Check sheet for the modelled part. Datum: model origin and axes. Units: mm. A direction names the side the tool comes from. Round coordinates to 2 decimals unless told otherwise and drop trailing zeros. Loops run counter-clockwise (first coordinate to the right, second up) from the corner with the lowest first, then second, coordinate; pieces in that order, holes last. Notation, with made-up numbers: (-24, -11.75) - (-5, -11.75) arc R34 ccw to (-5, 22.25) - close; hole circle Ø5 at (-33.75, 3.5). An arc over 180 degrees is marked (long way). Put each result on its own line as item: value.
```python
from build123d import *

# Parameters (mm, degrees)
EXTRUDE_1_DEPTH     = 10
SKETCH_2_W          = 16
SKETCH_2_H          = 40
CUT_EXTRUDE_1_DEPTH = 10
SKETCH_3_R          = 2
CUT_EXTRUDE_2_DEPTH = 50


with BuildPart() as part:
    # 草图1 → 凸台-拉伸1 (new, symmetric)
    with BuildSketch(Plane.XY):
        Polygon((0, 42), (0, 2), (0, 0), (7, 0), (7, 44), (0, 44), align=None)
    extrude(amount=EXTRUDE_1_DEPTH, both=True)

    # 草图2 → 切除-拉伸1 (cut, symmetric)
    with BuildSketch(Plane(origin=(7, 0, 0), x_dir=(0, 0, -1), z_dir=(1, 0, 0))):
        with Locations((0, 22)):
            Rectangle(SKETCH_2_W, SKETCH_2_H)
    extrude(amount=CUT_EXTRUDE_1_DEPTH, both=True, mode=Mode.SUBTRACT)

    # 草图3 → 切除-拉伸2 (cut)
    with BuildSketch(Plane(origin=(0, 44, 0), x_dir=(1, 0, 0), z_dir=(0, 1, 0))):
        with Locations(Location((4, 5, 0), (0, 0, 270))):
            Circle(SKETCH_3_R)
        with Locations(Location((4, -5, 0), (0, 0, 270))):
            Circle(SKETCH_3_R)
    extrude(amount=-CUT_EXTRUDE_2_DEPTH, mode=Mode.SUBTRACT)


solid = part.part
```
Item 1: Section check C-C on z = -1.5. Enter the section's corners in (x, y).
Filled sheet:
outline: (0, 0) - (7, 0) - (7, 2) - (0, 2) - close; (0, 42) - (7, 42) - (7, 44) - (0, 44) - close
Item 2: Release check for a two-part mould opening along Y. For faces 1 (the flat face through (4, 44, 0)), 2 (the flat face through (3, 22, -10)), 3 (the flat face through (4, 42, 0)) record: +Y half, -Y half, draft (parallel to the pull), parting line (faces both ways), or undercut.
Filled sheet:
face 1: +Y half
face 2: draft
face 3: undercut
Item 3: Thickness scan on line 1 (Y direction, x = 1.25, z = -3.75); line 2 (Z direction, x = 1, y = 17); line 3 (X direction, y = 0.65, z = 5). Record the ranges inside material, lowest first. Write a range as from..to.
Filled sheet:
line 1: 0..2, 42..44
line 2: -10..-8, 8..10
line 3: 0..2, 6..7
Item 4: Section check B-B on x = 6.5. Enter the section's corners in (y, z), then the cut area to 3 significant figures.
Filled sheet:
outline: (0, -10) - (44, -10) - (44, 10) - (0, 10) - close; hole (2, -8) - (42, -8) - (42, 8) - (2, 8) - close
area: 240 mm²
Item 5: Section check D-D on x = 4. Enter the section's corners in (y, z).
Filled sheet:
outline: (0, -10) - (44, -10) - (44, -7) - (42, -7) - (42, -8) - (2, -8) - (2, -7) - (0, -7) - close; (0, -3) - (2, -3) - (2, 3) - (0, 3) - close; (0, 7) - (2, 7) - (2, 8) - (42, 8) - (42, 7) - (44, 7) - (44, 10) - (0, 10) - close; (42, -3) - (44, -3) - (44, 3) - (42, 3) - close
Item 6: Section check A-A on z = 5. Enter the section's corners in (x, y).
Filled sheet:
outline: (0, 0) - (2, 0) - (2, 2) - (0, 2) - close; (0, 42) - (2, 42) - (2, 44) - (0, 44) - close; (6, 0) - (7, 0) - (7, 2) - (6, 2) - close; (6, 42) - (7, 42) - (7, 44) - (6, 44) - close
Item 7: Tool access check on faces 4 (the flat face through (4, 2, 0)), 5 (the flat face through (3, 0, 0)). Record the directions out of +Z, -Z, +X, -X, +Y, -Y that give a thin tool (end or side, any length) a straight path to the whole face; none if there is none.
Filled sheet:
face 4: +X, -X
face 5: +Z, -Z, +X, -X, -Y
Item 8: Go/stop test with a flat-tipped pin: pin 1 (2 mm diameter, centred on y = 15.5, z = 6, fed in from -X). Record where the tip stops, or that it passes through.
Filled sheet:
pin 1: through
